```python
from build123d import *

# Parameters (mm, degrees)
F0_W          = 67
F0_H          = 138
F1_DEPTH      = 7
F2_T          = -2
F4_DEPTH      = 2
F6_DEPTH      = 2
F8_DEPTH      = 2
F10_D         = 5
F10_DEPTH     = 2
F10_TIP       = 1.5021515476
F11_T1_DEPTH  = 135
F11_T3_DEPTH  = 64
F11_T5_DEPTH  = 4
F11_S9_W      = 1.5
F11_S9_H      = 1.5
F11_T10_DEPTH = 1.5
F11_S15_W     = 1.5
F11_S15_H     = 1.5
F11_T16_DEPTH = 1.5
F11_S21_W     = 1.5
F11_S21_H     = 1.5
F11_T22_DEPTH = 1.5
F11_S27_W     = 1.5
F11_S27_H     = 1.5
F11_T28_DEPTH = 1.5
F11_S33_W     = 1.5
F11_S33_H     = 1.5
F11_T34_DEPTH = 1.5
F11_S39_W     = 1.5
F11_S39_H     = 1.5
F11_T40_DEPTH = 1.5
F11_S45_W     = 1.5
F11_S45_H     = 1.5
F11_T46_DEPTH = 1.5
F11_S51_W     = 1.5
F11_S51_H     = 1.5
F11_T52_DEPTH = 1.5


# Not quite as in the source:
# - a fillet or chamfer that OpenCascade refuses, or shapes differently, is made with other operations: its cross-section is extruded or revolved along the edge and cut away or added


with BuildPart() as f1:
    # F0 (on Top) → F1 (new body)
    with BuildSketch(Plane.XY):
        Rectangle(F0_W, F0_H)
    extrude(amount=F1_DEPTH)

    # F2
    f2_openings = [f1.faces().sort_by_distance(p)[0] for p in [
        (0, 0, 7),
    ]]
    offset(amount=F2_T, openings=f2_openings)

    # F3 (on face) → F4 (cut, through all)
    with BuildSketch(Plane(origin=(-33.5, 0, 0), x_dir=(0, -1, 0), z_dir=(-1, 0, 0))):
        with BuildLine():
            Line((-22.538946541, 5), (-61.0191351455, 5))
            ThreePointArc((-61.0191351455, 5), (-61.5564696174, 4.7774287742), (-61.7790408432, 4.2400943022))
            Line((-61.7790408432, 4.2400943022), (-61.7790408432, 2.7599056978))
            ThreePointArc((-61.7790408432, 2.7599056978), (-61.5564696174, 2.2225712258), (-61.0191351455, 2))
            Line((-61.0191351455, 2), (-22.538946541, 2))
            ThreePointArc((-22.538946541, 2), (-22.0016120691, 2.2225712258), (-21.7790408432, 2.7599056978))
            Line((-21.7790408432, 2.7599056978), (-21.7790408432, 4.2400943022))
            ThreePointArc((-21.7790408432, 4.2400943022), (-22.0016120691, 4.7774287742), (-22.538946541, 5))
        make_face()
    extrude(amount=-F4_DEPTH, mode=Mode.SUBTRACT)

    # F5 (on face) → F6 (cut, through all)
    with BuildSketch(Plane.YZ.offset(33.5)):
        with BuildLine():
            Line((36.2400943022, 5), (24.7599056978, 5))
            ThreePointArc((24.7599056978, 5), (24.2225712258, 4.7774287742), (24, 4.2400943022))
            Line((24, 4.2400943022), (24, 2.7599056978))
            ThreePointArc((24, 2.7599056978), (24.2225712258, 2.2225712258), (24.7599056978, 2))
            Line((24.7599056978, 2), (36.2400943022, 2))
            ThreePointArc((36.2400943022, 2), (36.7774287742, 2.2225712258), (37, 2.7599056978))
            Line((37, 2.7599056978), (37, 4.2400943022))
            ThreePointArc((37, 4.2400943022), (36.7774287742, 4.7774287742), (36.2400943022, 5))
        make_face()
    extrude(amount=-F6_DEPTH, mode=Mode.SUBTRACT)

    # F7 (on face) → F8 (cut, through all)
    with BuildSketch(Plane.XZ.offset(69)):
        with BuildLine():
            Line((11.7400943022, 5), (-11.7400943022, 5))
            ThreePointArc((-11.7400943022, 5), (-12.2774287742, 4.7774287742), (-12.5, 4.2400943022))
            Line((-12.5, 4.2400943022), (-12.5, 2.7599056978))
            ThreePointArc((-12.5, 2.7599056978), (-12.2774287742, 2.2225712258), (-11.7400943022, 2))
            Line((-11.7400943022, 2), (11.7400943022, 2))
            ThreePointArc((11.7400943022, 2), (12.2774287742, 2.2225712258), (12.5, 2.7599056978))
            Line((12.5, 2.7599056978), (12.5, 4.2400943022))
            ThreePointArc((12.5, 4.2400943022), (12.2774287742, 4.7774287742), (11.7400943022, 5))
        make_face()
    extrude(amount=-F8_DEPTH, mode=Mode.SUBTRACT)

    # F10
    with Locations(Plane.XZ.offset(69)):
        with Locations((18.5, 3.5)):
            Hole(F10_D / 2, depth=F10_DEPTH)
            with Locations((0, 0, -(F10_DEPTH + F10_TIP / 2))):  # 118° drill point
                Cone(0, F10_D / 2, F10_TIP, mode=Mode.SUBTRACT)

    # F11: fillet of radius 1.5 on 12 edges, made by hand

    # F11_s2 → F11_t1 (cut)
    with BuildSketch(Plane.XZ.offset(-67.5)):
        with BuildLine():
            ThreePointArc((33.5, 5.5), (33.0606601718, 6.5606601718), (32, 7))
            Line((32, 7), (33.5, 7))
            Line((33.5, 7), (33.5, 5.5))
        make_face()
        with BuildLine():
            ThreePointArc((33.5, 1.5), (33.0606601718, 0.4393398282), (32, 0))
            Line((32, 0), (33.5, 0))
            Line((33.5, 0), (33.5, 1.5))
        make_face()
        with BuildLine():
            ThreePointArc((-32, 7), (-33.0606601718, 6.5606601718), (-33.5, 5.5))
            Line((-33.5, 5.5), (-33.5, 7))
            Line((-33.5, 7), (-32, 7))
        make_face()
        with BuildLine():
            ThreePointArc((-32, 0), (-33.0606601718, 0.4393398282), (-33.5, 1.5))
            Line((-33.5, 1.5), (-33.5, 0))
            Line((-33.5, 0), (-32, 0))
        make_face()
    extrude(amount=F11_T1_DEPTH, mode=Mode.SUBTRACT)

    # F11_s4 → F11_t3 (cut)
    with BuildSketch(Plane.YZ.offset(-32)):
        with BuildLine():
            ThreePointArc((-69, 5.5), (-68.5606601718, 6.5606601718), (-67.5, 7))
            Line((-67.5, 7), (-69, 7))
            Line((-69, 7), (-69, 5.5))
        make_face()
        with BuildLine():
            ThreePointArc((-69, 1.5), (-68.5606601718, 0.4393398282), (-67.5, 0))
            Line((-67.5, 0), (-69, 0))
            Line((-69, 0), (-69, 1.5))
        make_face()
        with BuildLine():
            ThreePointArc((67.5, 7), (68.5606601718, 6.5606601718), (69, 5.5))
            Line((69, 5.5), (69, 7))
            Line((69, 7), (67.5, 7))
        make_face()
        with BuildLine():
            ThreePointArc((67.5, 0), (68.5606601718, 0.4393398282), (69, 1.5))
            Line((69, 1.5), (69, 0))
            Line((69, 0), (67.5, 0))
        make_face()
    extrude(amount=F11_T3_DEPTH, mode=Mode.SUBTRACT)

    # F11_s6 → F11_t5 (cut)
    with BuildSketch(Plane.XY.offset(1.5)):
        with BuildLine():
            ThreePointArc((33.5, -67.5), (33.0606601718, -68.5606601718), (32, -69))
            Line((32, -69), (33.5, -69))
            Line((33.5, -69), (33.5, -67.5))
        make_face()
        with BuildLine():
            ThreePointArc((33.5, 67.5), (33.0606601718, 68.5606601718), (32, 69))
            Line((32, 69), (33.5, 69))
            Line((33.5, 69), (33.5, 67.5))
        make_face()
        with BuildLine():
            ThreePointArc((-32, 69), (-33.0606601718, 68.5606601718), (-33.5, 67.5))
            Line((-33.5, 67.5), (-33.5, 69))
            Line((-33.5, 69), (-32, 69))
        make_face()
        with BuildLine():
            ThreePointArc((-32, -69), (-33.0606601718, -68.5606601718), (-33.5, -67.5))
            Line((-33.5, -67.5), (-33.5, -69))
            Line((-33.5, -69), (-32, -69))
        make_face()
    extrude(amount=F11_T5_DEPTH, mode=Mode.SUBTRACT)


with BuildPart() as f11_tool8:
    # F11_s9 → F11_t10 (new body)
    with BuildSketch(Plane.YZ.offset(32)):
        with Locations((-68.25, 6.25)):
            Rectangle(F11_S9_W, F11_S9_H)
    extrude(amount=F11_T10_DEPTH)

    # F11_s11 → F11_t12 (revolve, cut)
    with BuildSketch(Plane(origin=(32, -67.5, 5.5), x_dir=(0, 0.7071067812, -0.7071067812), z_dir=(0, -0.7071067812, -0.7071067812))):
        with BuildLine():
            ThreePointArc((0, -1.5), (1.5, 0), (0, 1.5))
            Line((0, 1.5), (0, -1.5))
        make_face()
    revolve(axis=Axis((32, -67.5, 5.5), (1, 0, 0)), mode=Mode.SUBTRACT)


with BuildPart() as f1_1:
    add(f1.part)

    # F11_t7: cut F11_tool8
    add(f11_tool8.part, mode=Mode.SUBTRACT)


with BuildPart() as f11_tool14:
    # F11_s15 → F11_t16 (new body)
    with BuildSketch(Plane.YZ.offset(32)):
        with Locations((68.25, 6.25)):
            Rectangle(F11_S15_W, F11_S15_H)
    extrude(amount=F11_T16_DEPTH)

    # F11_s17 → F11_t18 (revolve, cut)
    with BuildSketch(Plane(origin=(32, 67.5, 5.5), x_dir=(0, -0.7071067812, -0.7071067812), z_dir=(0, -0.7071067812, 0.7071067812))):
        with BuildLine():
            ThreePointArc((0, -1.5), (1.5, 0), (0, 1.5))
            Line((0, 1.5), (0, -1.5))
        make_face()
    revolve(axis=Axis((32, 67.5, 5.5), (1, 0, 0)), mode=Mode.SUBTRACT)


with BuildPart() as f1_2:
    add(f1_1.part)

    # F11_t13: cut F11_tool14
    add(f11_tool14.part, mode=Mode.SUBTRACT)


with BuildPart() as f11_tool20:
    # F11_s21 → F11_t22 (new body)
    with BuildSketch(Plane.XZ.offset(67.5)):
        with Locations((-32.75, 6.25)):
            Rectangle(F11_S21_W, F11_S21_H)
    extrude(amount=F11_T22_DEPTH)

    # F11_s23 → F11_t24 (revolve, cut)
    with BuildSketch(Plane(origin=(-32, -67.5, 5.5), x_dir=(0.7071067812, 0, -0.7071067812), z_dir=(-0.7071067812, 0, -0.7071067812))):
        with BuildLine():
            ThreePointArc((0, -1.5), (1.5, 0), (0, 1.5))
            Line((0, 1.5), (0, -1.5))
        make_face()
    revolve(axis=Axis((-32, -67.5, 5.5), (0, -1, 0)), mode=Mode.SUBTRACT)


with BuildPart() as f1_3:
    add(f1_2.part)

    # F11_t19: cut F11_tool20
    add(f11_tool20.part, mode=Mode.SUBTRACT)


with BuildPart() as f11_tool26:
    # F11_s27 → F11_t28 (new body)
    with BuildSketch(Plane.XZ.offset(67.5)):
        with Locations((-32.75, 0.75)):
            Rectangle(F11_S27_W, F11_S27_H)
    extrude(amount=F11_T28_DEPTH)

    # F11_s29 → F11_t30 (revolve, cut)
    with BuildSketch(Plane(origin=(-32, -67.5, 1.5), x_dir=(0.7071067812, 0, 0.7071067812), z_dir=(0.7071067812, 0, -0.7071067812))):
        with BuildLine():
            ThreePointArc((0, -1.5), (1.5, 0), (0, 1.5))
            Line((0, 1.5), (0, -1.5))
        make_face()
    revolve(axis=Axis((-32, -67.5, 1.5), (0, -1, 0)), mode=Mode.SUBTRACT)


with BuildPart() as f1_4:
    add(f1_3.part)

    # F11_t25: cut F11_tool26
    add(f11_tool26.part, mode=Mode.SUBTRACT)


with BuildPart() as f11_tool32:
    # F11_s33 → F11_t34 (new body)
    with BuildSketch(Plane.YZ.offset(32)):
        with Locations((-68.25, 0.75)):
            Rectangle(F11_S33_W, F11_S33_H)
    extrude(amount=F11_T34_DEPTH)

    # F11_s35 → F11_t36 (revolve, cut)
    with BuildSketch(Plane(origin=(32, -67.5, 1.5), x_dir=(0, 0.7071067812, 0.7071067812), z_dir=(0, 0.7071067812, -0.7071067812))):
        with BuildLine():
            ThreePointArc((0, -1.5), (1.5, 0), (0, 1.5))
            Line((0, 1.5), (0, -1.5))
        make_face()
    revolve(axis=Axis((32, -67.5, 1.5), (1, 0, 0)), mode=Mode.SUBTRACT)


with BuildPart() as f1_5:
    add(f1_4.part)

    # F11_t31: cut F11_tool32
    add(f11_tool32.part, mode=Mode.SUBTRACT)


with BuildPart() as f11_tool38:
    # F11_s39 → F11_t40 (new body)
    with BuildSketch(Plane.YZ.offset(32)):
        with Locations((68.25, 0.75)):
            Rectangle(F11_S39_W, F11_S39_H)
    extrude(amount=F11_T40_DEPTH)

    # F11_s41 → F11_t42 (revolve, cut)
    with BuildSketch(Plane(origin=(32, 67.5, 1.5), x_dir=(0, -0.7071067812, 0.7071067812), z_dir=(0, 0.7071067812, 0.7071067812))):
        with BuildLine():
            ThreePointArc((0, -1.5), (1.5, 0), (0, 1.5))
            Line((0, 1.5), (0, -1.5))
        make_face()
    revolve(axis=Axis((32, 67.5, 1.5), (1, 0, 0)), mode=Mode.SUBTRACT)


with BuildPart() as f1_6:
    add(f1_5.part)

    # F11_t37: cut F11_tool38
    add(f11_tool38.part, mode=Mode.SUBTRACT)


with BuildPart() as f11_tool44:
    # F11_s45 → F11_t46 (new body)
    with BuildSketch(Plane.XY.offset(5.5)):
        with Locations((-32.75, 68.25)):
            Rectangle(F11_S45_W, F11_S45_H)
    extrude(amount=F11_T46_DEPTH)

    # F11_s47 → F11_t48 (revolve, cut)
    with BuildSketch(Plane(origin=(-32, 67.5, 5.5), x_dir=(0.7071067812, -0.7071067812, 0), z_dir=(-0.7071067812, -0.7071067812, 0))):
        with BuildLine():
            ThreePointArc((0, -1.5), (1.5, 0), (0, 1.5))
            Line((0, 1.5), (0, -1.5))
        make_face()
    revolve(axis=Axis((-32, 67.5, 5.5), (0, 0, 1)), mode=Mode.SUBTRACT)


with BuildPart() as f1_7:
    add(f1_6.part)

    # F11_t43: cut F11_tool44
    add(f11_tool44.part, mode=Mode.SUBTRACT)


with BuildPart() as f11_tool50:
    # F11_s51 → F11_t52 (new body)
    with BuildSketch(Plane.XY.offset(1.5)):
        with Locations((-32.75, 68.25)):
            Rectangle(F11_S51_W, F11_S51_H)
    extrude(amount=-F11_T52_DEPTH)

    # F11_s53 → F11_t54 (revolve, cut)
    with BuildSketch(Plane(origin=(-32, 67.5, 1.5), x_dir=(0.7071067812, -0.7071067812, 0), z_dir=(0.7071067812, 0.7071067812, 0))):
        with BuildLine():
            ThreePointArc((0, -1.5), (1.5, 0), (0, 1.5))
            Line((0, 1.5), (0, -1.5))
        make_face()
    revolve(axis=Axis((-32, 67.5, 1.5), (0, 0, -1)), mode=Mode.SUBTRACT)


with BuildPart() as f1_8:
    add(f1_7.part)

    # F11_t49: cut F11_tool50
    add(f11_tool50.part, mode=Mode.SUBTRACT)


solid = f1_8.part
```
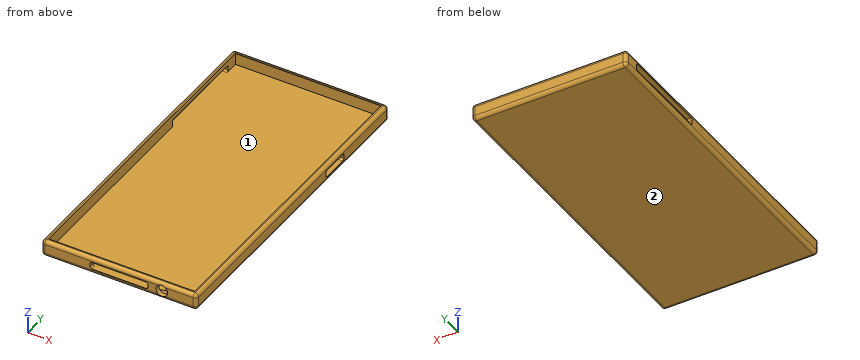
Verification items for the finished model (mm, model axes). Face numbers are marked on the shaded views. Coordinates: 2 decimals unless noted, no trailing zeros. Loops run counter-clockwise (first coordinate to the right, second up) from the corner with the lowest first, then second, coordinate; pieces in that order, holes last. Notation, with made-up numbers: (-6, -13.5) - (0, -13.5) arc R15 cw to (0, -0.5) - close; hole circle Ø5 at (68.25, 57.25). An arc over 180 degrees is marked (long way). Return JSON: item names as keys, results as strings.
1. Thickness scan on L1, parallel to X at y = -67.45, z = 3.5; L2, parallel to Y at x = 13.5, z = 5.5; L3, parallel to X at y = -40.5, z = 5.25. Record the ranges inside material, lowest first.
Established:
{"L1": "x = -33.5 to -12.5, 12.5 to 16, 21 to 33.5", "L2": "y = -69 to -67, 67 to 69", "L3": "x = -33.5 to -31.5, 31.5 to 33.5"}
2. Section check C-C, the plane y = 3. Record the boundary of the cut face in (x, z).
Established:
{"outline": "(-33.5, 1.5) arc R1.5 ccw to (-32, 0) - (32, 0) arc R1.5 ccw to (33.5, 1.5) - (33.5, 5.5) arc R1.5 ccw to (32, 7) - (31.5, 7) - (31.5, 2) - (-31.5, 2) - (-31.5, 7) - (-32, 7) arc R1.5 ccw to (-33.5, 5.5) - close"}
3. Section check B-B, the plane x = -28. Record the boundary of the cut face in (y, z), then the cut area to 3 significant figures.
Established:
{"outline": "(-69, 1.5) arc R1.5 ccw to (-67.5, 0) - (67.5, 0) arc R1.5 ccw to (69, 1.5) - (69, 5.5) arc R1.5 ccw to (67.5, 7) - (67, 7) - (67, 2) - (-67, 2) - (-67, 7) - (-67.5, 7) arc R1.5 ccw to (-69, 5.5) - close", "area": "294 mm2"}
4. Go/stop test with flat-tipped pins: pin 1 (1 mm diameter, centred on y = -52.5, z = 6, fed in from -X); pin 2 (1.2 mm diameter, centred on x = -33, z = 3.5, fed in from +Y); pin 3 (0.6 mm diameter, centred on x = 33, y = 30, fed in from -Z); pin 4 (8 mm diameter, centred on x = 18, y = -49, fed in from +Z). Record where each tip stops, or that it passes through.
Established:
{"pin 1": "stops at x = -33.5", "pin 2": "stops at y = 68.95", "pin 3": "stops at z = 0.17", "pin 4": "stops at z = 2"}
5. Section check D-D, the plane x = 18.5. Record the boundary of the cut face in (y, z), then the cut area to 3 significant figures.
Established:
{"outline": "(-68.91, 1) arc R1.5 ccw to (-67.5, 0) - (67.5, 0) arc R1.5 ccw to (69, 1.5) - (69, 5.5) arc R1.5 ccw to (67.5, 7) - (67, 7) - (67, 2) - (-66.4, 2) - (-67, 1) - close; (-68.91, 6) - (-67, 6) - (-67, 7) - (-67.5, 7) arc R1.5 ccw to start", "area": "284 mm2"}
6. Section check A-A, the plane x = 5. Record the boundary of the cut face in (y, z), then the cut area to 3 significant figures.
Established:
{"outline": "(-69, 1.5) arc R1.5 ccw to (-67.5, 0) - (67.5, 0) arc R1.5 ccw to (69, 1.5) - (69, 5.5) arc R1.5 ccw to (67.5, 7) - (67, 7) - (67, 2) - (-69, 2) - close; (-69, 5) - (-67, 5) - (-67, 7) - (-67.5, 7) arc R1.5 ccw to (-69, 5.5) - close", "area": "288 mm2"}
7. Mould release check, pull along Y, two halves, no side actions. Record for the marked faces 1 and 2: +Y half, -Y half, draft (parallel to the pull), parting line (faces both ways), or undercut.
Established:
{"face 1": "undercut", "face 2": "draft"}
